from build123d import *

# Parameters (mm, degrees)
CHANFREIN3_SIZE         = 1
ENL_V_MAT_EXTRU_1_DEPTH = 44.852023899
CHANFREIN1_SIZE         = 1
CHANFREIN2_SIZE         = 0.5


with BuildPart() as part:
    # Esquisse1 → Révolution1 (revolve)
    with BuildSketch(Plane.XY, mode=Mode.PRIVATE) as r_volution1_sk:
        Polygon((4.8, 10), (4, 10), (4, 26), (5.2, 26), (5.2, 32), (6.5, 32), (6.5, 41), (11, 41), (11, 25), (9.55, 25), (9.55, 26.13), (7.55, 26.13), (7.55, 25), (7, 25), (7, 0), (4.8, 0), align=None)
    revolve(r_volution1_sk.sketch.rotate(Axis((0, 0, 0), (0, 1, 0)), 90), axis=Axis((0, 0, 0), (0, 1, 0)))

    # Chanfrein3
    chanfrein3_edges = [part.edges().sort_by_distance(p)[0] for p in [
        (0, 41, 11),
    ]]
    chamfer(chanfrein3_edges, length=CHANFREIN3_SIZE)

    # Esquisse2 → Enlèv. mat.-Extru.1 (cut, through all)
    with BuildSketch(Plane(origin=(0, 41, 0), x_dir=(1, 0, 0), z_dir=(0, 1, 0))):
        with BuildLine():
            Line((-10, 4.582575695), (-10, -4.582575695))
            ThreePointArc((-10, -4.582575695), (-11, 0), (-10, 4.582575695))
        make_face()
        with BuildLine():
            Line((10, 4.582575695), (10, -4.582575695))
            ThreePointArc((10, -4.582575695), (11, 0), (10, 4.582575695))
        make_face()
    extrude(amount=-ENL_V_MAT_EXTRU_1_DEPTH, mode=Mode.SUBTRACT)

    # Chanfrein1
    chanfrein1_edges = [part.edges().sort_by_distance(p)[0] for p in [
        (0, 41, 6.5),
        (0, 0, 7),
    ]]
    chamfer(chanfrein1_edges, length=CHANFREIN1_SIZE)

    # Chanfrein2
    chanfrein2_edges = [part.edges().sort_by_distance(p)[0] for p in [
        (0, 10, 4),
        (0, 26, 4),
        (0, 32, 5.2),
        (0, 0, 4.8),
    ]]
    chamfer(chanfrein2_edges, length=CHANFREIN2_SIZE)


solid = part.part
Model file for the job. Use its own axes, mm. A direction names the side the tool comes from. Give positions to 0.01 mm unless a question says otherwise; leave off trailing zeros. Loops run counter-clockwise (first coordinate to the right, second up) from the corner with the lowest first, then second, coordinate; pieces in that order, holes last.
Item 1: Drop flat-ended pins along their axis: P1, Ø8.5, axis at x = 1, z = 2.5, coming from the +Y side; P2, Ø3, axis at y = 27.5, z = 5.5, coming from the +X side; P3, Ø6.5, axis at x = 0, z = 0, coming from the +Y side; P4, Ø1.5, axis at x = -7.5, z = 8.5, coming from the -Y side. Give the stop position or say it passes through.
Check values:
P1: stops at y = 40.44
P2: stops at x = 10
P3: passes through
P4: stops at y = 25
Item 2: Slice it at C-C (y = 12.5). Write the cut outline in (x, z), plus the area to 3 significant figures.
Check values:
outline: circle Ø14 at (0, 0); hole circle Ø8 at (0, 0)
area: 104 mm2
Item 3: Mould opens along X. For faces 1 (the face through (-0.2, 40.8, 10.2)), 2 (the face through (-10, 33, 0)), 3 (the face through (10, 33, 0)), 4 (the face through (-8, 26.13, -1)) say: +X half, -X half, draft (parallel to the pull), parting line (faces both ways), or undercut.
Check values:
face 1: parting line
face 2: -X half
face 3: +X half
face 4: undercut
Item 4: Drill centre lines: line 1 along X through (y, z) = (25.3, 0); line 2 along X through (y, z) = (6.25, 0); line 3 along X through (y, z) = (20.5, 0). Where is each one in solid material? Low to high.
Check values:
line 1: x = -10 to -9.55, -7.55 to -4, 4 to 7.55, 9.55 to 10
line 2: x = -7 to -4.8, 4.8 to 7
line 3: x = -7 to -4, 4 to 7
Item 5: Which spindle directions (+Z, -Z, +X, -X, +Y, -Y) get a long thin tool onto all of the face, cutting with end or side? Do faces 5 (the face through (7.37, 25.56, 1.64)), 6 (the face through (0.2, 40.8, -10.2)). Say none if no direction does.
Check values:
face 5: -Y
face 6: -Z, +Y
Item 6: Slice it at B-B (y = 38). Write the cut outline in (x, z).
Check values:
outline: (-10, -4.58) arc R11 ccw to (10, -4.58) - (10, 4.58) arc R11 ccw to (-10, 4.58) - close; hole circle Ø13 at (0, 0)
Item 7: Slice it at A-A (y = 27). Write the cut outline in (x, z).
Check values:
outline: (-10, -4.58) arc R11 ccw to (10, -4.58) - (10, 4.58) arc R11 ccw to (-10, 4.58) - close; hole circle Ø10.4 at (0, 0)
